```python
from build123d import *

# Parameters (mm, degrees)
SKETCH1_W           = 30
SKETCH1_H           = 19
SKETCH1_W_2         = 24
SKETCH1_H_2         = 13
BOSS_EXTRUDE1_DEPTH = 5
BOSS_EXTRUDE4_DEPTH = 4
SKETCH4_W           = 6
SKETCH4_H           = 19
BOSS_EXTRUDE5_DEPTH = 6
LPATTERN1_COUNT     = 2
LPATTERN1_PITCH     = 79
SKETCH6_W           = 12
SKETCH6_H           = 19
BOSS_EXTRUDE6_DEPTH = 5
LPATTERN2_COUNT     = 2
LPATTERN2_PITCH     = 73
BOSS_EXTRUDE7_DEPTH = 3
FILLET1_R           = 1
FILLET2_R           = 1
FILLET3_R           = 1


with BuildPart() as part:
    # Sketch1 → Boss-Extrude1 (new body)
    with BuildSketch(Plane.XY):
        with Locations((12, 6.5)):
            Rectangle(SKETCH1_W, SKETCH1_H)
        with Locations((12, 6.5)):
            Rectangle(SKETCH1_W_2, SKETCH1_H_2, mode=Mode.SUBTRACT)
    extrude(amount=BOSS_EXTRUDE1_DEPTH)

    # Sketch3 → Boss-Extrude4 (add)
    with BuildSketch(Plane(origin=(0, 0, 0), x_dir=(-1, 0, 0), z_dir=(0, 0, -1))):
        Polygon((-12, 16), (-54.5, 16), (-54.5, -3), (-7, -3), (30.5, -3), (30.5, 16), align=None)
    extrude(amount=BOSS_EXTRUDE4_DEPTH)

    # Sketch4 → Boss-Extrude5 (add)
    with BuildSketch(Plane(origin=(0, 0, -4), x_dir=(-1, 0, 0), z_dir=(0, 0, -1))):
        with Locations((-51.5, 6.5)):
            Rectangle(SKETCH4_W, SKETCH4_H)
    boss_extrude5 = extrude(amount=BOSS_EXTRUDE5_DEPTH)

    # LPattern1: Boss-Extrude5 ×2
    with Locations(*[(-i * LPATTERN1_PITCH, 0, 0) for i in range(1, LPATTERN1_COUNT)]):
        add(boss_extrude5)

    # Sketch6 → Boss-Extrude6 (add)
    with BuildSketch(Plane(origin=(0, 0, -10), x_dir=(-1, 0, 0), z_dir=(0, 0, -1))):
        with Locations((-48.5, 6.5)):
            Rectangle(SKETCH6_W, SKETCH6_H)
    boss_extrude6 = extrude(amount=BOSS_EXTRUDE6_DEPTH)

    # LPattern2: Boss-Extrude6 ×2
    with Locations(*[(-i * LPATTERN2_PITCH, 0, 0) for i in range(1, LPATTERN2_COUNT)]):
        add(boss_extrude6)

    # Sketch7 → Boss-Extrude7 (add)
    with BuildSketch(Plane.XY.offset(5)):
        Polygon((12, 0), (7, 0), (7, -3), (12, -3), (17, -3), (17, 0), align=None)
    extrude(amount=BOSS_EXTRUDE7_DEPTH)

    # Fillet1
    fillet1_edges = [part.edges().sort_by_distance(p)[0] for p in [
        (-3, 16, 2.5),
        (27, 16, 2.5),
        (27, -3, 2.5),
        (-3, -3, 2.5),
    ]]
    fillet(fillet1_edges, radius=FILLET1_R)

    # Fillet2
    fillet2_edges = [part.edges().sort_by_distance(p)[0] for p in [
        (54.5, 16, -7.5),
        (54.5, -3, -7.5),
        (-30.5, -3, -7.5),
        (-30.5, 16, -7.5),
    ]]
    fillet(fillet2_edges, radius=FILLET2_R)

    # Fillet3
    fillet3_edges = [part.edges().sort_by_distance(p)[0] for p in [
        (48.5, 6.5, -4),
        (48.5, 6.5, -10),
        (-24.5, 6.5, -4),
        (-24.5, 6.5, -10),
    ]]
    fillet(fillet3_edges, radius=FILLET3_R)


solid = part.part
```
The listing builds one solid part. Answer for the finished solid, in the listing's coordinates (mm). A direction names the side the tool comes from. Round coordinates to 2 decimals unless told otherwise and drop trailing zeros. Order: outer loops, then holes, each group sorted by start corner. A loop starts at its lowest first (then second) coordinate and runs counter-clockwise, first axis right, second up. Notation, with made-up numbers: (63, 38) - (89, 38) arc R34 cw to (89, 70) - close; hole circle Ø11 at (55, 58). An arc over 180 degrees is marked (long way). Put each result on its own line as item: value. Start each with the question number.
(1) For faces 4 (the flat face through (12, 7, 0)), 5 (the flat face through (45, 7, -10)), 6 (the flat face through (11, 14, 5)), 7 (the flat face through (7, -1, 6)), determine the directions among +Z, -Z, +X, -X, +Y, -Y from which every point of the face is accessible in a straight line to the end or side of a thin tool.
(2) Find section B-B (x = 46.5). Give the vertices of the cut face in (y, z), plus the area to 3 significant figures.
(3) Given P1, Ø5.5, axis at x = 36.5, y = 4.5, coming from the +Z side; P2, Ø1, axis at x = 30, y = 10.5, coming from the -Z side; P3, Ø1.5, axis at y = -1.5, z = 6.5, coming from the +X side, each flat-ended and moving along its own axis, determine where each tip first touches the part or whether it passes through.
(4) Find section A-A (z = -8). Give the vertices of the cut face in (x, y).
(5) Find section C-C (z = 1.25). Give the vertices of the cut face in (x, y).
(6) Find section D-D (y = 0.75). Give the vertices of the cut face in (x, z).
(7) Determine the mould class of faces 1 (the flat face through (0, 6, 2)), 2 (the flat face through (-16, 7, 0)), 3 (the flat face through (13, -3, -3)) for opening direction Y: released by +Y, released by -Y, zero draft, split by the parting line, or undercut.
(8) Straight lines are drawn through the part: probe 1 along X at (y, z) = (-1.5, -10.25); probe 2 along X at (y, z) = (14.75, -8.25); probe 3 along X at (y, z) = (-1.5, 3). For each, find the intervals that lie inside material, in ascending order. Write a range as from..to.
Reply:
1. face 4: +Z
1. face 5: +Y, -Y
1. face 6: +Z, +Y
1. face 7: +Z, -X, +Y, -Y
2. outline: (-3, -15) - (16, -15) - (16, -10) - (-3, -10) - close; (-3, -4) - (16, -4) - (16, 0) - (-3, 0) - close
2. area: 171 mm^2
3. P1: z = 0
3. P2: z = -4
3. P3: x = 17
4. outline: (-30.5, -2) arc R1 ccw to (-29.5, -3) - (-24.5, -3) - (-24.5, 16) - (-29.5, 16) arc R1 ccw to (-30.5, 15) - close; (48.5, -3) - (53.5, -3) arc R1 ccw to (54.5, -2) - (54.5, 15) arc R1 ccw to (53.5, 16) - (48.5, 16) - close
5. outline: (-3, -2) arc R1 ccw to (-2, -3) - (26, -3) arc R1 ccw to (27, -2) - (27, 15) arc R1 ccw to (26, 16) - (-2, 16) arc R1 ccw to (-3, 15) - close; hole (0, 0) - (24, 0) - (24, 13) - (0, 13) - close
6. outline: (-30.5, -15) - (-18.5, -15) - (-18.5, -10) - (-23.5, -10) arc R1 cw to (-24.5, -9) - (-24.5, -5) arc R1 cw to (-23.5, -4) - (47.5, -4) arc R1 cw to (48.5, -5) - (48.5, -9) arc R1 cw to (47.5, -10) - (42.5, -10) - (42.5, -15) - (54.5, -15) - (54.5, 0) - (27, 0) - (27, 5) - (24, 5) - (24, 0) - (0, 0) - (0, 5) - (-3, 5) - (-3, 0) - (-30.5, 0) - close
7. face 1: undercut
7. face 2: zero draft
7. face 3: released by -Y
8. probe 1: -30.5..-18.5, 42.5..54.5
8. probe 2: -30.5..-24.5, 48.5..54.5
8. probe 3: -3..27
